Work out the finished part from the listing and answer in its coordinate system (mm). Coordinates: 2 decimals unless noted, no trailing zeros. Write each loop counter-clockwise with the first axis right and the second up, starting at its lowest first coordinate (ties: lowest second). Pieces come first, ordered by that corner, then holes. Notation, with made-up numbers: M -9,-17.5 L 44,-17.5 A34 ccw 44,16.5 Z; hole C 44.25,81 d5. An arc over 180 degrees is marked long. Answer as CSV lines item,"result". Start each with the question number.
(1) Find the intervals of material crossed by L1, parallel to X at y = 0.85, z = 15.5; L2, parallel to X at y = 1.75, z = -31.5; L3, parallel to Z at x = 13, y = 0.5, in increasing order. Write a range as [from, to].
(2) A flat-ended cylindrical pin translates along its axis: P1, Ø3, axis at x = -13, z = -31.5, coming from the -Y side. Find the tip coordinate at first contact, or state that the pin passes through.
(3) A cutting plane is placed at C-C on y = 1.3. Give the vertices of the cut face in (x, z) (3 decimals).
(4) A cutting plane is placed at A-A on x = -12. Give the vertices of the cut face in (y, z) (3 decimals).
(5) A cutting plane is placed at B-B on z = -9. Give the vertices of the cut face in (x, y) (3 decimals), then the cut area to 3 significant figures.
(6) A cutting plane is placed at D-D on z = -31.5. Give the vertices of the cut face in (x, y) (3 decimals), then the cut area to 3 significant figures.
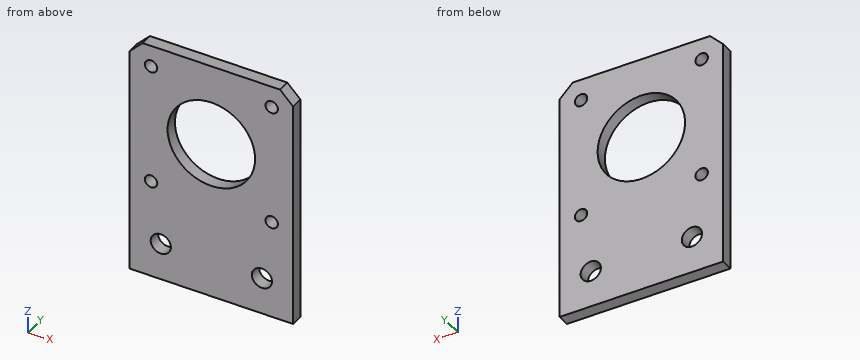
from build123d import *

# Parameters (mm, degrees)
SKETCH1_R           = 2.6
SKETCH1_R_2         = 1.6
SKETCH1_R_3         = 11.25
BOSS_EXTRUDE1_DEPTH = 3.175


with BuildPart() as part:
    # Sketch1 → Boss-Extrude1 (new body)
    with BuildSketch(Plane(origin=(0, 0, 0), x_dir=(1, 0, 0), z_dir=(0, 1, 0))):
        Polygon((21, 41), (-21, 41), (-21, 17.645), (-17.645, 21), (17.645, 21), (21, 17.645), align=None)
        with Locations((-13, 31.5)):
            Circle(SKETCH1_R, mode=Mode.SUBTRACT)
        with Locations((13, 31.5)):
            Circle(SKETCH1_R, mode=Mode.SUBTRACT)
        Polygon((-21, -17.645), (-21, 17.645), (-17.645, 21), (17.645, 21), (21, 17.645), (21, -17.645), (17.645, -21), (-17.645, -21), align=None)
        with Locations((15.5, -15.5)):
            Circle(SKETCH1_R_2, mode=Mode.SUBTRACT)
        with Locations((15.5, 15.5)):
            Circle(SKETCH1_R_2, mode=Mode.SUBTRACT)
        with Locations((-15.5, 15.5)):
            Circle(SKETCH1_R_2, mode=Mode.SUBTRACT)
        with Locations((-15.5, -15.5)):
            Circle(SKETCH1_R_2, mode=Mode.SUBTRACT)
        Circle(SKETCH1_R_3, mode=Mode.SUBTRACT)
    extrude(amount=BOSS_EXTRUDE1_DEPTH)


solid = part.part
Here are the results:
1,L1,"x = [-21, -17.1], [-13.9, 13.9], [17.1, 21]"
1,L2,"x = [-21, -15.6], [-10.4, 10.4], [15.6, 21]"
1,L3,"z = [-41, -34.1], [-28.9, 21]"
2,P1,"passes through"
3,outline,"M -21,-41 L 21,-41 L 21,17.645 L 17.645,21 L -17.645,21 L -21,17.645 Z; hole C -15.5,-15.5 d3.2; hole C -15.5,15.5 d3.2; hole C -13,-31.5 d5.2; hole C 0,0 d22.5; hole C 13,-31.5 d5.2; hole C 15.5,-15.5 d3.2; hole C 15.5,15.5 d3.2"
4,outline,"M 0,-41 L 3.175,-41 L 3.175,-33.9 L 0,-33.9 Z; M 0,-29.1 L 3.175,-29.1 L 3.175,21 L 0,21 Z"
5,outline,"M -21,0 L -6.75,0 L -6.75,3.175 L -21,3.175 Z; M 6.75,0 L 21,0 L 21,3.175 L 6.75,3.175 Z"
5,area,"90.5 mm^2"
6,outline,"M -21,0 L -15.6,0 L -15.6,3.175 L -21,3.175 Z; M -10.4,0 L 10.4,0 L 10.4,3.175 L -10.4,3.175 Z; M 15.6,0 L 21,0 L 21,3.175 L 15.6,3.175 Z"
6,area,"100 mm^2"
